Check sheet for the modelled part. Datum: model origin and axes. Units: mm. Coordinates: 2 decimals unless noted, no trailing zeros. Use CSV: the item, a comma, the result in double quotes. Start each with the question number.
(1) Draft check along Z on faces 1 (the flat face through (-4.96, -8.59, 15.93)), 2 (the cylindrical face through (0.62, -15, 21.43)). Enter one of: pulls with the +Z half, pulls with the -Z half, needs draft (parallel to the pull), parting line crosses it, or undercut.
(2) Go/stop test with flat-tipped pins: pin 1 Ø5 at (y, z) = (-12, 22.5) entering from +X; pin 2 Ø5 at (x, z) = (6, 0.5) entering from +Y; pin 3 Ø10 at (x, y) = (-8.5, -24) entering from +Z. Record where each tip stops, or that it passes through.
(3) Scan lines: line 1 (Z direction, x = -1, y = -15); line 2 (Z direction, x = 4, y = -22); line 3 (Y direction, x = -8, z = 16.5). Record each from-to range of solid material in increasing order.
from build123d import *

# Parameters (mm, degrees)
F1_ANGLE_BACK = 30
F1_ANGLE      = 60
F2_R          = 4.5079852031
F3_DEPTH      = 15
F4_R          = 2


with BuildPart() as f1:
    # F0 (on Right) → F1 (revolve)
    with BuildSketch(Plane.YZ, mode=Mode.PRIVATE) as f1_sk:
        with BuildLine():
            Line((0, 0), (0, 27))
            add(Edge.make_bspline(
                [(0, 27), (-5.5034394129, 32.661690712), (-15.8471030498, 59.3621170559), (-10.5280846021, 19.7077828646), (-41.0819364315, 33.8046592086), (-10.5991049383, 16.215764014), (-29.7721432902, -5.3374961203), (-4.7977967218, 12.3670629457), (-5.5203058645, -16.1073831097), (-1.4451971006, -4.7678385339), (0, 0)],
                knots=[0, 0, 0, 0, 0.150530903, 0.287029044, 0.4059261233, 0.5423978305, 0.661868087, 0.7802364409, 0.9001627782, 1, 1, 1, 1], degree=3))
        make_face()
    revolve(f1_sk.sketch.rotate(Axis((0, 0, 13.5), (0, 0, -1)), -F1_ANGLE_BACK), axis=Axis((0, 0, 13.5), (0, 0, -1)), revolution_arc=F1_ANGLE)

    # F2 (on face) → F3 (cut, symmetric)
    with BuildSketch(Plane(origin=(0, 0, 0), x_dir=(-0.5, 0.8660254038, 0), z_dir=(0.8660254038, 0.5, 0))):
        with Locations((-9.7265727818, 24.1762548685)):
            Circle(F2_R)
    extrude(amount=F3_DEPTH, both=True, mode=Mode.SUBTRACT)

    # F4
    f4_edges = [f1.edges().sort_by_distance(p)[0] for p in [
        (7.117279, -12.327489, 24.176255),
    ]]
    fillet(f4_edges, radius=F4_R)


solid = f1.part
Outcome:
1,face 1,"needs draft"
1,face 2,"undercut"
2,pin 1,"stops at x = 8.37"
2,pin 2,"stops at y = -16.52"
2,pin 3,"stops at z = 28.54"
3,line 1,"z = 4.05 to 20.61, 27.74 to 30.22"
3,line 2,"z = 1 to 2.31, 20.94 to 26.64"
3,line 3,"y = -17.73 to -13.86"
